Could you check a few things on this drawing? It's one solid part, dimensions in mm from its lowest x, y, z. A direction names the side the tool comes from. Give positions to 0.01 mm unless a question says otherwise; leave off trailing zeros. Loops run counter-clockwise (first coordinate to the right, second up) from the corner with the lowest first, then second, coordinate; pieces in that order, holes last. Notation, with made-up numbers: M -17.75,-28 L 37.25,-28 A18 cw 37.25,5 Z; hole C 43.5,-10 d7. An arc over 180 degrees is marked long. Answer in a Markdown table with one row per item. Add a question column.
1. I need wall thicknesses on line 1 along Y through (x, z) = (7.25, 0.7) (1 decimal); line 2 along Y through (x, z) = (6.5, 4.1) (1 decimal); line 3 along Z through (x, y) = (7.5, 7.5). Which ranges of each line are inside material? Lowest first, please. Write a range as from..to.
2. If we section it at A-A on x = 8: List the corners of the cut face in (y, z) for me.
3. Which directions (+Z, -Z, +X, -X, +Y, -Y) give clear straight access to the entire face, cutting with the end or side of a thin tool? Please do the marked faces 1 and 2.
4. Thinking about a two-plate mould opening in X: for the marked faces 3, 4 and 5, which applies, released by +X, released by -X, zero draft, split by the parting line, or undercut?
5. If we section it at C-C on z = 3.25: List the corners of the cut face in (x, y) for me.
6. If we section it at D-D on x = 14: List the corners of the cut face in (y, z) for me.
7. I'm going to push flat-ended pins straight in: pin 1 Ø2 at (x, y) = (11.5, 47.5) entering from -Z; pin 2 Ø2 at (x, z) = (5.5, 2) entering from +Y; pin 3 Ø0.9 at (x, y) = (10.97, 48.17) entering from +Z. Where does each tip first touch, or does it pass through?
8. If we section it at B-B on y = 12: List the corners of the cut face in (x, z) for me (1 decimal).
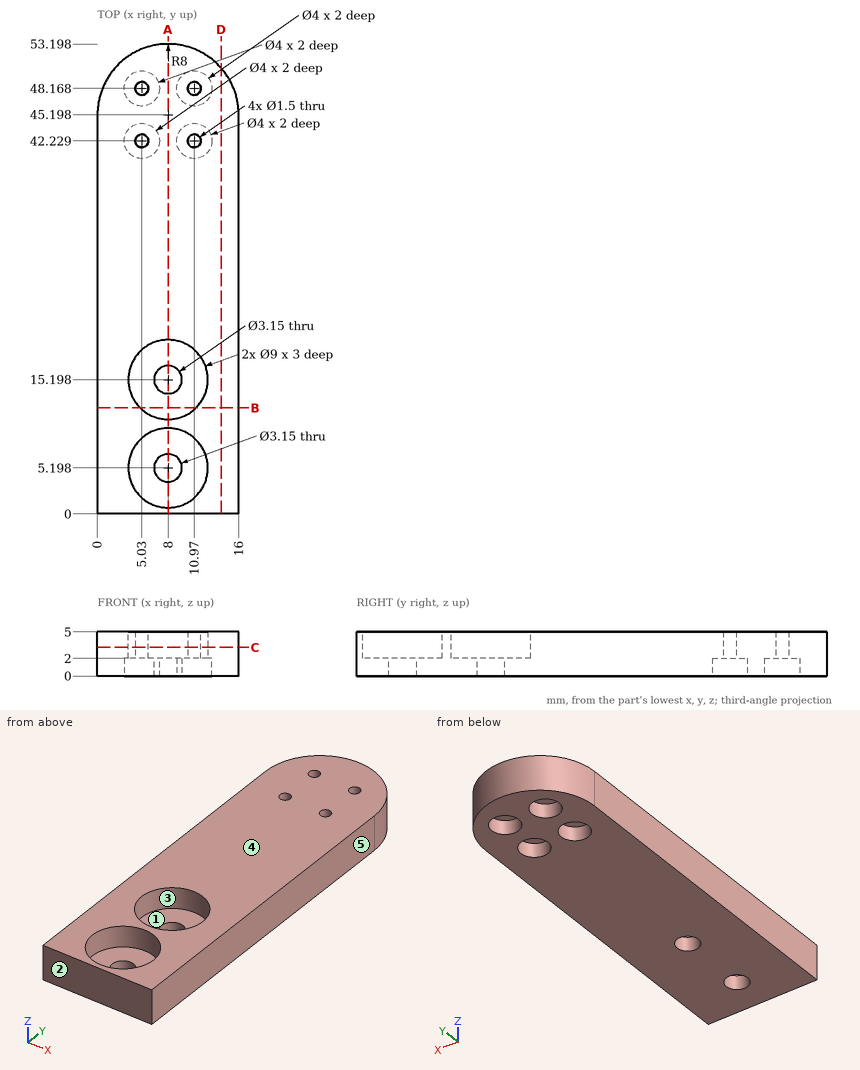
Results:
| question | item | result |
|---|---|---|
| 1 | line 1 | 0..3.8, 6.6..13.8, 16.6..53.2 |
| 1 | line 2 | 0..1, 9.4..11, 19.4..53.1 |
| 1 | line 3 | 0..2 |
| 2 | outline | M 0,0 L 3.62,0 L 3.62,2 L 0.7,2 L 0.7,5 L 0,5 Z; M 6.77,0 L 13.62,0 L 13.62,2 L 10.7,2 L 10.7,5 L 9.7,5 L 9.7,2 L 6.77,2 Z; M 16.77,0 L 53.2,0 L 53.2,5 L 19.7,5 L 19.7,2 L 16.77,2 Z |
| 3 | face 1 | +Z |
| 3 | face 2 | +Z, -Z, +X, -X, -Y |
| 4 | face 3 | undercut |
| 4 | face 4 | zero draft |
| 4 | face 5 | released by +X |
| 5 | outline | M 0,0 L 16,0 L 16,45.2 A8 ccw 0,45.2 Z; hole C 8,5.2 d9; hole C 8,15.2 d9; hole C 5.03,42.23 d1.5; hole C 5.03,48.17 d1.5; hole C 10.97,42.23 d1.5; hole C 10.97,48.17 d1.5 |
| 6 | outline | M 0,0 L 50.49,0 L 50.49,5 L 0,5 Z |
| 7 | pin 1 | z = 2 |
| 7 | pin 2 | y = 53.06 |
| 7 | pin 3 | through |
| 8 | outline | M 0,0 L 16,0 L 16,5 L 11.2,5 L 11.2,2 L 4.8,2 L 4.8,5 L 0,5 Z |
